For this review, take the finished solid that the model builds, in its own axes (mm). A direction names the side the tool comes from. Give positions to 0.01 mm unless a question says otherwise; leave off trailing zeros. Loops run counter-clockwise (first coordinate to the right, second up) from the corner with the lowest first, then second, coordinate; pieces in that order, holes last.
```python
from build123d import *

# Parameters (mm, degrees)
EXTRUDE_1_DEPTH        = 10
HOLE_WIZARD_M8_1_D     = 6.8
HOLE_WIZARD_M8_1_DEPTH = 19.75
HOLE_WIZARD_M8_1_TIP   = 2.042926105


with BuildPart() as part:
    # 草图1 → 凸台-拉伸1 (new, symmetric)
    with BuildSketch(Plane.XY):
        with BuildLine():
            Line((4, -9.6), (-4, -9.6))
            ThreePointArc((-4, -9.6), (-7.592990245, -7.621309711), (-10, -4.3))
            Line((-10, -4.3), (-10, -3.3))
            Line((-10, -3.3), (-4, -3.3))
            Line((-4, -3.3), (-4, 0))
            Line((-4, 0), (4, 0))
            Line((4, 0), (4, -3.3))
            Line((4, -3.3), (10, -3.3))
            Line((10, -3.3), (10, -4.3))
            ThreePointArc((10, -4.3), (7.592990245, -7.621309711), (4, -9.6))
        make_face()
    extrude(amount=EXTRUDE_1_DEPTH, both=True)

    # M8 螺纹孔1
    with Locations(Plane.ZX):
        with Locations((0, 0)):
            Hole(HOLE_WIZARD_M8_1_D / 2, depth=HOLE_WIZARD_M8_1_DEPTH)
            with Locations((0, 0, -(HOLE_WIZARD_M8_1_DEPTH + HOLE_WIZARD_M8_1_TIP / 2))):  # 118° drill point
                Cone(0, HOLE_WIZARD_M8_1_D / 2, HOLE_WIZARD_M8_1_TIP, mode=Mode.SUBTRACT)


solid = part.part
```
Item 1: Take a section at D-D on y = -1.5. Give the boundary of the cut face in (x, z), and give its area (3 significant figures).
Answer:
outline: (-4, -10) - (4, -10) - (4, 10) - (-4, 10) - close; hole circle Ø6.8 at (0, 0)
area: 124 mm2
Item 2: Take a section at C-C on z = 7.5. Give the boundary of the cut face in (x, y), and give its area (3 significant figures).
Answer:
outline: (-10, -4.3) arc R9.39 ccw to (-4, -9.6) - (4, -9.6) arc R9.39 ccw to (10, -4.3) - (10, -3.3) - (4, -3.3) - (4, 0) - (-4, 0) - (-4, -3.3) - (-10, -3.3) - close
area: 130 mm2
Item 3: Tool access review of faces 1 (the flat face through (0, -6, 10)), 2 (the flat face through (4, -2, 0)), 3 (the flat face through (-4, -2, 0)): name each direction out of +Z, -Z, +X, -X, +Y, -Y from which nothing blocks a thin tool from reaching the whole face with its end or side.
Answer:
face 1: +Z, +X, -X, +Y, -Y
face 2: +Z, -Z, +X, +Y
face 3: +Z, -Z, -X, +Y
Item 4: For L1, parallel to X at y = -3.25, z = 0; L2, parallel to X at y = -5.75, z = 0; L3, parallel to X at y = -1.25, z = 6.5, list the stretches that pass through material, from the lowest coordinate up.
Answer:
L1: x = -4 to -3.4, 3.4 to 4
L2: x = -9.22 to -3.4, 3.4 to 9.22
L3: x = -4 to 4
Item 5: Take a section at B-B on z = 0. Give the boundary of the cut face in (x, y), and give its area (3 significant figures).
Answer:
outline: (-10, -4.3) arc R9.39 ccw to (-4, -9.6) - (-3.4, -9.6) - (-3.4, 0) - (-4, 0) - (-4, -3.3) - (-10, -3.3) - close; (3.4, -9.6) - (4, -9.6) arc R9.39 ccw to (10, -4.3) - (10, -3.3) - (4, -3.3) - (4, 0) - (3.4, 0) - close
area: 65.0 mm2
Item 6: Clearance check with flat-ended pins moving along their axes: pin 1 Ø1.6 at (y, z) = (-2, 2) entering from -X; pin 2 Ø8 at (x, z) = (0, 0) entering from -Y; pin 3 Ø5 at (x, z) = (-7, -2) entering from -Y; pin 4 Ø2.5 at (y, z) = (-2, -3) entering from +X. State where each tip first meets the part, or that it passes through.
Answer:
pin 1: stops at x = -4
pin 2: stops at y = -9.6
pin 3: stops at y = -9.44
pin 4: stops at x = 4
Item 7: The part is to be moulded in two halves that separate along X. For faces 4 (the cylindrical face through (7.64, -7.58, 0.14)), 5 (the flat face through (-10, -4, 0)), 6 (the cylindrical face through (-3.32, -4.87, 0.74)), 7 (the flat face through (0, -6, -10)), say which applies: released by +X, released by -X, zero draft, split by the parting line, or undercut.
Answer:
face 4: released by +X
face 5: released by -X
face 6: undercut
face 7: zero draft
Item 8: Take a section at A-A on x = 0. Give the boundary of the cut face in (y, z), and give its area (3 significant figures).
Answer:
outline: (-9.6, -10) - (0, -10) - (0, -3.4) - (-9.6, -3.4) - close; (-9.6, 3.4) - (0, 3.4) - (0, 10) - (-9.6, 10) - close
area: 127 mm2
